```python
from build123d import *

# Parameters (mm, degrees)
F0_W      = 52
F0_H      = 56.2
F1_DEPTH  = 4
F2_W      = 52
F2_H      = 56.2
F3_DEPTH  = 17.5
F5_DEPTH  = 1
F6_R      = 3.25
F7_DEPTH  = 2
F9_DEPTH  = 2.6
F10_R     = 1.65
F11_DEPTH = 21.501
F12_R     = 2
F13_R     = 1


with BuildPart() as f1:
    # F0 (on Top) → F1 (new body)
    with BuildSketch(Plane.XY):
        with Locations((26, 28.1)):
            Rectangle(F0_W, F0_H)
    extrude(amount=F1_DEPTH)

    # F2 (on face) → F3 (join)
    with BuildSketch(Plane.XY.offset(4)):
        with Locations((26, 28.1)):
            Rectangle(F2_W, F2_H)
        Polygon((2, 2), (2, 54.2), (50, 54.2), (50, 2), (23.8, 2), (23.8, 48.2), (21.8, 48.2), (21.8, 2), align=None, mode=Mode.SUBTRACT)
    extrude(amount=F3_DEPTH)

    # F4 (on face) → F5 (cut)
    with BuildSketch(Plane.XY.offset(4)):
        Polygon((2.6, 45.881166), (2.6, 22.581166), (7.6, 17.262331), (14.9, 17.262331), (19.9, 22.581166), (19.9, 45.881166), (14.9, 51.2), (7.6, 51.2), align=None)
    extrude(amount=-F5_DEPTH, mode=Mode.SUBTRACT)

    # F6 (on face) → F7 (cut, through all)
    with BuildSketch(Plane.YZ.offset(2)):
        with Locations((8.75, 12.75)):
            Circle(F6_R)
    extrude(amount=-F7_DEPTH, mode=Mode.SUBTRACT)

    # F8 (on face) → F9 (cut)
    with BuildSketch(Plane(origin=(0, 0, 0), x_dir=(1, 0, 0), z_dir=(0, 0, -1))):
        Polygon((19.9, -10.022947), (22.8, -11.697263), (25.7, -10.022947), (25.7, -6.674316), (22.8, -5), (19.9, -6.674316), align=None)
        Polygon((22.8, -44.502737), (19.9, -46.177053), (19.9, -49.525684), (22.8, -51.2), (25.7, -49.525684), (25.7, -46.177053), align=None)
    extrude(amount=-F9_DEPTH, mode=Mode.SUBTRACT)

    # F10 (on face) → F11 (cut, through all)
    with BuildSketch(Plane(origin=(0, 0, 0), x_dir=(1, 0, 0), z_dir=(0, 0, -1))):
        with Locations((22.8, -47.851368)):
            Circle(F10_R)
        with Locations((22.8, -8.348632)):
            Circle(F10_R)
    extrude(amount=-F11_DEPTH, mode=Mode.SUBTRACT)

    # F12
    f12_edges = [f1.edges().sort_by_distance(p)[0] for p in [
        (0, 0, 10.75),
        (52, 0, 10.75),
        (0, 56.2, 10.75),
        (52, 56.2, 10.75),
    ]]
    fillet(f12_edges, radius=F12_R)

    # F13
    f13_edges = [f1.edges().sort_by_distance(p)[0] for p in [
        (50, 54.2, 12.75),
        (50, 2, 12.75),
        (2, 2, 12.75),
        (2, 54.2, 12.75),
        (21.8, 2, 12.75),
        (23.8, 2, 12.75),
    ]]
    fillet(f13_edges, radius=F13_R)


solid = f1.part
```
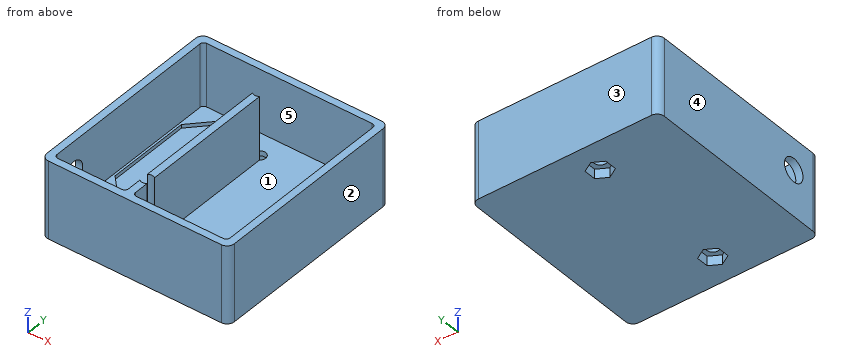
Can you work these out from the model? Positions are in its coordinate system, mm. Face numbers are marked on the shaded views. A direction names the side the tool comes from. Coordinates: 2 decimals unless noted, no trailing zeros. Loops run counter-clockwise (first coordinate to the right, second up) from the corner with the lowest first, then second, coordinate; pieces in that order, holes last.
1) Imagine slicing it at B-B on y = 41. List the corners of the cut face in (x, z) for me, plus the area to 3 significant figures.
2) Imagine slicing it at C-C on x = 14. List the corners of the cut face in (y, z) for me, plus the area to 3 significant figures.
3) Imagine slicing it at D-D on y = 9. List the corners of the cut face in (x, z) for me, plus the area to 3 significant figures.
4) Which directions (+Z, -Z, +X, -X, +Y, -Y) give clear straight access to the entire face, cutting with the end or side of a thin tool? Please do the marked faces 1 and 2.
5) Thinking about a two-plate mould opening in X: for the marked faces 3, 4 and 5, which applies, pulls with the +X half, pulls with the -X half, needs draft (parallel to the pull), parting line crosses it, or undercut?
6) I need wall thicknesses on probe 1 along Y at (x, z) = (22.8, 15.75); probe 2 along X at (y, z) = (5.5, 19); probe 3 along Y at (x, z) = (12, 15.25). Which ranges of each line are inside material? Lowest first, please.
7) For pin 1 (5 mm diameter, centred on x = 38.5, y = 16.5, fed in from +Z); pin 2 (8.5 mm diameter, centred on x = 12.5, y = 37.5, fed in from +Z); pin 3 (3 mm diameter, centred on x = 23, y = 48.5, fed in from -Z), each with a flat end and sliding along its axis, tell me the tip position at first contact or that it passes through.
Completed:
1. outline: (0, 0) - (52, 0) - (52, 21.5) - (50, 21.5) - (50, 4) - (23.8, 4) - (23.8, 21.5) - (21.8, 21.5) - (21.8, 4) - (19.9, 4) - (19.9, 3) - (2.6, 3) - (2.6, 4) - (2, 4) - (2, 21.5) - (0, 21.5) - close
1. area: 296 mm2
2. outline: (0, 0) - (56.2, 0) - (56.2, 21.5) - (54.2, 21.5) - (54.2, 4) - (51.2, 4) - (51.2, 3) - (17.26, 3) - (17.26, 4) - (2, 4) - (2, 21.5) - (0, 21.5) - close
2. area: 261 mm2
3. outline: (0, 0) - (19.9, 0) - (19.9, 2.6) - (21.28, 2.6) - (21.28, 4) - (2, 4) - (2, 9.51) - (0, 9.51) - close; (0, 15.99) - (2, 15.99) - (2, 21.5) - (0, 21.5) - close; (24.32, 2.6) - (25.7, 2.6) - (25.7, 0) - (52, 0) - (52, 21.5) - (50, 21.5) - (50, 4) - (24.32, 4) - close
3. area: 246 mm2
4. face 1: +Z
4. face 2: +Z, -Z, +X, +Y, -Y
5. face 3: needs draft
5. face 4: pulls with the -X half
5. face 5: undercut
6. probe 1: y = 0 to 6.7, 10 to 46.2, 54.2 to 56.2
6. probe 2: x = 0 to 2, 21.8 to 23.8, 50 to 52
6. probe 3: y = 0 to 2, 54.2 to 56.2
7. pin 1: stops at z = 4
7. pin 2: stops at z = 3
7. pin 3: stops at z = 2.6
